```python
from build123d import *

# Parameters (mm, degrees)
SKETCH2_W           = 30
SKETCH2_H           = 10
BOSS_EXTRUDE3_DEPTH = 6
CUT_EXTRUDE2_DEPTH  = 4
SKETCH5_W           = 30
SKETCH5_H           = 10
CUT_EXTRUDE3_DEPTH  = 33.186953879
SKETCH6_R           = 1.5
CUT_EXTRUDE4_DEPTH  = 31.574253478
SKETCH7_R           = 0.75
CUT_EXTRUDE5_DEPTH  = 31.245412474


with BuildPart() as part:
    # Sketch2 → Boss-Extrude3 (new body)
    with BuildSketch(Plane(origin=(0, 0, 0), x_dir=(1, 0, 0), z_dir=(0, 1, 0))):
        with Locations((15, 5)):
            Rectangle(SKETCH2_W, SKETCH2_H)
    extrude(amount=BOSS_EXTRUDE3_DEPTH)

    # Sketch3 → Cut-Extrude2 (cut)
    with BuildSketch(Plane(origin=(0, 6, 0), x_dir=(1, 0, 0), z_dir=(0, 1, 0))):
        with BuildLine():
            Line((6.127698587, 1.42357778), (20.75, 2.9))
            ThreePointArc((20.75, 2.9), (22.85, 5), (20.75, 7.1))
            Line((20.75, 7.1), (6.45010187, 8.45828058))
            ThreePointArc((6.45010187, 8.45828058), (1.253932106, 5.171683811), (6.127698587, 1.42357778))
        make_face()
    extrude(amount=-CUT_EXTRUDE2_DEPTH, mode=Mode.SUBTRACT)

    # Sketch5 → Cut-Extrude3 (cut, through all)
    with BuildSketch(Plane(origin=(0, 6, 0), x_dir=(1, 0, 0), z_dir=(0, 1, 0))):
        with Locations((15, 5)):
            Rectangle(SKETCH5_W, SKETCH5_H)
        with BuildLine():
            Line((20.801973147, 8.099564291), (25.849999572, 7.501628842))
            ThreePointArc((25.849999572, 7.501628842), (28.349999572, 5.001628842), (25.849999572, 2.501628842))
            Line((25.849999572, 2.501628842), (20.805230344, 1.900492038))
            Line((20.805230344, 1.900492038), (6.324314639, 0.438345614))
            ThreePointArc((6.324314639, 0.438345614), (0.25385432, 5.191314364), (6.687176675, 9.440262928))
            Line((6.687176675, 9.440262928), (20.801973147, 8.099564291))
        make_face(mode=Mode.SUBTRACT)
    extrude(amount=-CUT_EXTRUDE3_DEPTH, mode=Mode.SUBTRACT)

    # Sketch6 → Cut-Extrude4 (cut, through all)
    with BuildSketch(Plane(origin=(0, 6, 0), x_dir=(1, 0, 0), z_dir=(0, 1, 0))):
        with Locations(Location((25.849999572, 5.001628842, 0), (0, 0, 270))):
            Circle(SKETCH6_R)
    extrude(amount=-CUT_EXTRUDE4_DEPTH, mode=Mode.SUBTRACT)

    # Sketch7 → Cut-Extrude5 (cut, through all)
    with BuildSketch(Plane(origin=(0, 2, 0), x_dir=(1, 0, 0), z_dir=(0, 1, 0))):
        with Locations(Location((5, 5, 0), (0, 0, 270))):
            Circle(SKETCH7_R)
    extrude(amount=-CUT_EXTRUDE5_DEPTH, mode=Mode.SUBTRACT)


solid = part.part
```
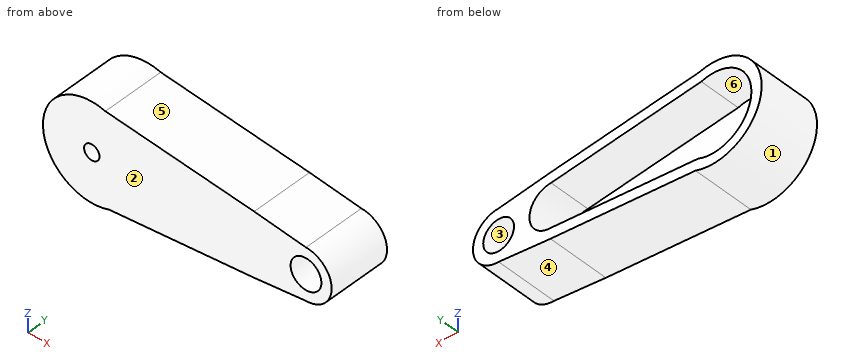
Input: part model. Units: mm. Frame: model coordinates. Face numbers are marked on the shaded views. A direction names the side the tool comes from. Round coordinates to 2 decimals unless told otherwise and drop trailing zeros. Loops run counter-clockwise (first coordinate to the right, second up) from the corner with the lowest first, then second, coordinate; pieces in that order, holes last. Notation, with made-up numbers: (25.5, 52) -> (81.5, 52) arc R21 ccw to (81.5, 57) -> close; hole circle Ø11 at (-38.75, 19.25). An arc over 180 degrees is marked (long way). Use one line per item in the form item = value. Start each with the question number.
Item 1: Section query D-D on z = -2.25. Return the cut outline in (x, y).
Item 2: Material intervals for L1, parallel to X at y = 5.1, z = -5; L2, parallel to X at y = 0.6, z = -5; L3, parallel to Z at x = 25.85, y = 3.55, sorted ascending. Write a range as from..to.
Item 3: Contact query for flat-ended pins moving along their axis: pin 1 Ø2 at (x, y) = (12, 4) entering from +Z; pin 2 Ø2 at (x, y) = (11, 3.5) entering from -Z; pin 3 Ø3 at (x, y) = (24.5, 1) entering from +Z; pin 4 Ø5 at (x, z) = (9, -5) entering from -Y. Output: stop coordinate, or through.
Item 4: Mould query, pull axis X, two halves, no side actions, for the marked faces 1, 2, 3 and 4. Classes: pulls with the +X half, pulls with the -X half, needs draft (parallel to the pull), parting line crosses it, or undercut.
Item 5: Section query C-C on y = 5.75. Return the cut outline in (x, z).
Item 6: Set-up query: the marked faces 5 and 6. Return all of +Z, -Z, +X, -X, +Y, -Y with unobstructed straight access to the full face (end or side cutting, diameter ignored); none if empty.
Item 7: Section query B-B on z = -5. Return the cut outline in (x, y), then the cut area to 3 significant figures.
Item 8: Section query A-A on x = 5. Return the cut outline in (y, z).
Ans:
q1.outline = (1.13, 0) -> (23.74, 0) -> (23.74, 6) -> (14.31, 6) -> (14.31, 2) -> (2.45, 2) -> (2.45, 6) -> (1.13, 6) -> close
q2.L1 = 0.25..1.25, 22.85..24.35, 27.35..28.35
q2.L2 = 0.25..4.25, 5.75..24.35, 27.35..28.35
q2.L3 = -7.5..-6.5, -3.5..-2.5
q3.pin_1 = -0.91
q3.pin_2 = -9.13
q3.pin_3 = -2.16
q3.pin_4 = 0
q4.face_1 = parting line crosses it
q4.face_2 = needs draft
q4.face_3 = undercut
q4.face_4 = pulls with the +X half
q5.outline = (6.32, -0.44) arc R4.75 ccw (long way) to (6.69, -9.44) -> (20.8, -8.1) -> (25.85, -7.5) arc R2.5 ccw to (25.85, -2.5) -> (20.81, -1.9) -> close; hole (6.13, -1.42) arc R3.75 ccw (long way) to (6.45, -8.46) -> (20.75, -7.1) arc R2.1 ccw to (20.75, -2.9) -> close; hole circle Ø3 at (25.85, -5)
q6.face_5 = +Z, +X, +Y, -Y
q6.face_6 = +Y
q7.outline = (0.25, 0) -> (4.25, 0) -> (4.25, 2) -> (1.25, 2) -> (1.25, 6) -> (0.25, 6) -> close; (5.75, 0) -> (24.35, 0) -> (24.35, 6) -> (22.85, 6) -> (22.85, 2) -> (5.75, 2) -> close; (27.35, 0) -> (28.35, 0) -> (28.35, 6) -> (27.35, 6) -> close
q7.area = 61.2 mm^2
q8.outline = (0, -9.75) -> (6, -9.75) -> (6, -8.75) -> (2, -8.75) -> (2, -5.75) -> (0, -5.75) -> close; (0, -4.25) -> (2, -4.25) -> (2, -1.25) -> (6, -1.25) -> (6, -0.25) -> (0, -0.25) -> close
